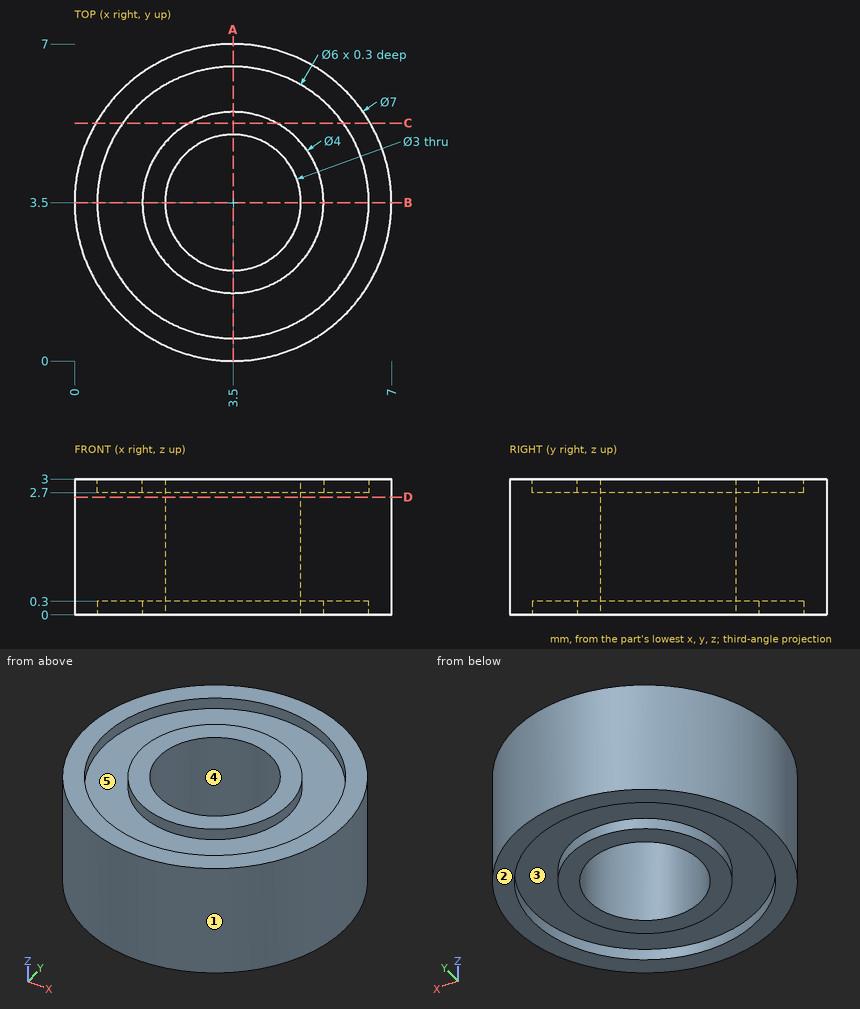
Could you check a few things on this drawing? It's one solid part, dimensions in mm from its lowest x, y, z. A direction names the side the tool comes from. Coordinates: 2 decimals unless noted, no trailing zeros. Order: outer loops, then holes, each group sorted by start corner. A loop starts at its lowest first (then second) coordinate and runs counter-clockwise, first axis right, second up. Notation, with made-up numbers: M -4.75,8.5 L 52.25,8.5 A29 cw 52.25,38.5 Z; hole C -9,25 d9. An arc over 180 degrees is marked long. Answer as a JSON object with one key per item and string values. Group by question number.
(1) Suppose I cut it at C-C, the plane y = 5.25. Please give me the cut outline in (x, z).
(2) I need wall thicknesses on probe 1 along Y at (x, z) = (3.5, 0.15); probe 2 along Y at (x, z) = (3.5, 2.4); probe 3 along X at (y, z) = (4.75, 0.1). Which ranges of each line are inside material? Lowest first, please.
(3) Which directions (+Z, -Z, +X, -X, +Y, -Y) give clear straight access to the entire face, cutting with the end or side of a thin tool? Please do the marked faces 4 and 5.
(4) For pin 1 (1.8 mm diameter, centred on x = 3.5, y = 4.5, fed in from -Z); pin 2 (1 mm diameter, centred on x = 5.5, z = 0.5, fed in from -Y), each with a flat end and sliding along its axis, tell me the tip position at first contact or that it passes through.
(5) Suppose I cut it at D-D, the plane z = 2.6. Please give me the cut outline in (x, y).
(6) Suppose I cut it at A-A, the plane x = 3.5. Please give me the cut outline in (y, z), then the cut area to 3 significant figures.
(7) If we mould it in two halves opening along X, with no side actions, what happens to the marked faces 1, 2 and 3? For each: released by +X, released by -X, zero draft, split by the parting line, or undercut.
Values found:
{
 "1": {"outline": "M 0.47,0 L 1.06,0 L 1.06,0.3 L 2.53,0.3 L 2.53,0 L 4.47,0 L 4.47,0.3 L 5.94,0.3 L 5.94,0 L 6.53,0 L 6.53,3 L 5.94,3 L 5.94,2.7 L 4.47,2.7 L 4.47,3 L 2.53,3 L 2.53,2.7 L 1.06,2.7 L 1.06,3 L 0.47,3 Z"},
 "2": {"probe 1": "y = 0 to 0.5, 1.5 to 2, 5 to 5.5, 6.5 to 7", "probe 2": "y = 0 to 2, 5 to 7", "probe 3": "x = 0.23 to 0.77, 1.94 to 2.67, 4.33 to 5.06, 6.23 to 6.77"},
 "3": {"face 4": "+Z, -Z", "face 5": "+Z"},
 "4": {"pin 1": "stops at z = 0", "pin 2": "stops at y = 0.34"},
 "5": {"outline": "C 3.5,3.5 d7; hole C 3.5,3.5 d3"},
 "6": {"outline": "M 0,0 L 0.5,0 L 0.5,0.3 L 1.5,0.3 L 1.5,0 L 2,0 L 2,3 L 1.5,3 L 1.5,2.7 L 0.5,2.7 L 0.5,3 L 0,3 Z; M 5,0 L 5.5,0 L 5.5,0.3 L 6.5,0.3 L 6.5,0 L 7,0 L 7,3 L 6.5,3 L 6.5,2.7 L 5.5,2.7 L 5.5,3 L 5,3 Z", "area": "10.8 mm^2"},
 "7": {"face 1": "split by the parting line", "face 2": "zero draft", "face 3": "undercut"}
}
